Autodesk Inventor part; units mm, degrees
ref_plane "Work Plane1" through (0, 0, 10) normal (0, 0, 1) x (1, 0, 0)
ref_plane "YZ Plane" through (0, 0, 0) normal (1, 0, 0) x (0, 1, 0)
ref_plane "XZ Plane" through (0, 0, 0) normal (0, 1, 0) x (-1, 0, 0)
ref_plane "Work Plane1" through (0, 0, 10) normal (0, 0, 1) x (1, 0, 0)
sketch "Sketch1" plane through (0, 0, 10) normal (0, 0, 1) x (1, 0, 0)
  line L0 (-4.0299, -0.3538) -> (-2.2322, 1.4439) construction
  arc A0 (-1.4439, 2.2322) -> (-2.2322, 1.4439) centre (-0.9299, 0.9299) ccw construction
  line L1 (-1.4439, 2.2322) -> (0.3538, 4.0299) construction
  line L2 (-37.8299, 42.2137) -> (-37.8299, 45.8299) construction
  line L3 (-37.8299, 45.8299) -> (-4.0299, 45.8299) construction
  line L4 (-4.0299, 45.8299) -> (-4.0299, 42.2137) construction
  line L5 (-4.0299, 4.0299) -> (0.3538, 4.0299)
  circle A1 centre (-20.9299, 20.9299) radius 17.5 construction
  line L6 (-20.9299, 58.9723) -> (17.1124, 20.9299) construction
  line L7 (17.1124, 20.9299) -> (-20.9299, -17.1124) construction
  line L8 (-20.9299, -17.1124) -> (-58.9723, 20.9299) construction
  line L9 (-58.9723, 20.9299) -> (-20.9299, 58.9723) construction
  line L10 (-20.9299, 58.9723) -> (-20.9299, -17.1124) construction
  line L11 (17.1124, 20.9299) -> (-58.9723, 20.9299) construction
  line L12 (-20.9299, 58.9723) -> (32.8701, 58.9723) construction
  line L13 (-43.2198, 43.4299) -> (1.7802, 43.4299) construction
  line L14 (1.7802, 43.4299) -> (1.7802, -1.5701) construction
  line L15 (1.7802, -1.5701) -> (-43.2198, -1.5701) construction
  line L16 (-43.2198, -1.5701) -> (-43.2198, 43.4299) construction
  line L17 (-43.2198, 5.1774) -> (-43.2198, 36.6824)
  line L18 (-43.2198, 36.6824) -> (-36.4723, 43.4299)
  line L19 (-36.4723, 43.4299) -> (-5.3876, 43.4299)
  line L20 (-5.3876, 43.4299) -> (1.7802, 36.2621)
  line L21 (1.7802, 36.2621) -> (1.7802, 5.5977)
  line L22 (1.7802, 5.5977) -> (-5.3876, -1.5701)
  line L23 (-5.3876, -1.5701) -> (-36.4723, -1.5701)
  line L24 (-36.4723, -1.5701) -> (-43.2198, 5.1774)
  line L25 (-4.0299, 42.2137) -> (-37.8299, 42.2137)
  line L26 (-4.0299, -0.3538) -> (-4.0299, 4.0299)
  circle A2 centre (-20.7198, 20.9299) radius 7.0417 construction
  arc A3 (-7.3745, 3.5) -> (-34.4854, 3.5) centre (-20.9299, 0) ccw construction
  arc A4 (-11.4668, 9.7661) -> (-30.4087, 10.1422) centre (-20.7198, 20.9299) ccw
  line L27 (-30.5806, 10.1422) -> (-30.4087, 10.1422)
  line L28 (-30.4087, 10.1422) -> (-30.4087, 1.6029)
  line L29 (-30.4087, 1.6029) -> (-11.4668, 1.6029)
  line L30 (-11.4668, 1.6029) -> (-11.4668, 9.7661)
  line L31 (-43.2198, 43.4299) -> (-10.4667, 10.6769) construction
  line L32 (-8.5595, 8.5517) -> (1.7802, -1.5701) construction
  line L33 (1.7802, 43.4299) -> (-25.699, 15.9507) construction
  line L34 (-30.9728, 10.6769) -> (-43.2198, -1.5701) construction
  point P0 (-37.8299, 4.0299)
  dimension "d18" = 53.8
  dimension "d19" = 45
  dimension "d20" = 53.8
  dimension "d21" = 45
  dimension "d22" = 45
  dimension "d68" = 29
extrude "Extrusion1" add sketch "Sketch1" along normal blind 8
sketch "Sketch3" plane through (0, 0, 10) normal (0, 0, -1) x (-1, 0, 0)
  line L0 (37.8299, -0.4701) -> (37.8299, 4.0299) construction
  line L1 (4.0299, 4.0299) -> (4.0299, -0.4701) construction
  line L2 (37.8299, -0.4701) -> (37.8299, 1.1886) construction
  line L3 (4.0299, -3.9701) -> (4.0299, -0.3538) construction
  line L4 (45.8299, 4.0299) -> (42.2137, 4.0299) construction
  line L5 (-0.3538, 4.0299) -> (-3.9701, 4.0299) construction
  line L6 (-3.9701, 37.8299) -> (-0.3538, 37.8299) construction
  line L7 (4.0299, 42.2137) -> (4.0299, 45.8299) construction
  line L8 (37.8299, 45.8299) -> (37.8299, 42.2137) construction
  line L9 (42.2137, 37.8299) -> (45.8299, 37.8299) construction
  line L10 (37.8299, 37.7299) -> (45.8299, 37.7299)
  line L11 (45.8299, 37.7299) -> (45.8299, 4.1299)
  line L12 (45.8299, 4.1299) -> (37.8299, 4.1299)
  line L13 (37.8299, 4.1299) -> (37.8299, 37.7299)
  line L14 (37.7299, 4.0299) -> (4.1299, 4.0299)
  line L15 (4.1299, 4.0299) -> (4.1299, -3.9701)
  line L16 (4.1299, -3.9701) -> (37.7299, -3.9701)
  line L17 (37.7299, -3.9701) -> (37.7299, 4.0299)
  line L18 (4.0299, 4.1299) -> (-3.9701, 4.1299)
  line L19 (-3.9701, 4.1299) -> (-3.9701, 37.7299)
  line L20 (-3.9701, 37.7299) -> (4.0299, 37.7299)
  line L21 (4.0299, 37.7299) -> (4.0299, 4.1299)
  line L22 (4.1299, 37.8299) -> (37.7299, 37.8299)
  line L23 (37.7299, 37.8299) -> (37.7299, 45.8299)
  line L24 (37.7299, 45.8299) -> (4.1299, 45.8299)
  line L25 (4.1299, 45.8299) -> (4.1299, 37.8299)
  point P0 (0, 0)
  dimension "d23" = 0.1
  dimension "d24" = 0.1
  dimension "d25" = 0.1
  dimension "d26" = 0.1
  dimension "d27" = 0.1
extrude "Extrusion3" add sketch "Sketch3" against normal up to surface (8 mm away)
sketch "Skizze12" plane through (0, 0, 10) normal (0, 0, -1) x (-1, 0, 0)
  line L0 (-0.3124, 4.1299) -> (4.1299, -0.3124)
  line L1 (4.1299, -0.3124) -> (4.1299, -3.9701)
  line L2 (4.1299, -3.9701) -> (37.7299, -3.9701) construction
  line L3 (37.7299, -3.9701) -> (37.7299, -0.3124)
  line L4 (37.7299, -0.3124) -> (42.1723, 4.1299)
  line L5 (45.8299, 4.1299) -> (42.1723, 4.1299)
  line L6 (45.8299, 37.7299) -> (45.8299, 4.1299) construction
  line L7 (42.1723, 37.7299) -> (45.8299, 37.7299)
  line L8 (42.1723, 37.7299) -> (37.7299, 42.1723)
  line L9 (37.7299, 42.1723) -> (37.7299, 45.8299)
  line L10 (37.7299, 45.8299) -> (4.1299, 45.8299) construction
  line L11 (4.1299, 45.8299) -> (4.1299, 42.1723)
  line L12 (4.1299, 42.1723) -> (-0.3124, 37.7299)
  line L13 (-3.9701, 37.7299) -> (-0.3124, 37.7299)
  line L14 (-3.9701, 4.1299) -> (-3.9701, 37.7299) construction
  line L15 (-0.3124, 4.1299) -> (-3.9701, 4.1299)
  line L16 (37.9299, -4.1701) -> (3.9299, -4.1701) construction
  line L17 (3.9299, -4.1701) -> (3.9299, -0.3953)
  line L18 (3.9299, -0.3953) -> (-0.3953, 3.9299)
  line L19 (-0.3953, 3.9299) -> (-4.1701, 3.9299)
  line L20 (-4.1701, 3.9299) -> (-4.1701, 37.9299) construction
  line L21 (-4.1701, 37.9299) -> (-0.3953, 37.9299)
  line L22 (-0.3953, 37.9299) -> (3.9299, 42.2551)
  line L23 (3.9299, 42.2551) -> (3.9299, 46.0299)
  line L24 (3.9299, 46.0299) -> (37.9299, 46.0299) construction
  line L25 (37.9299, 46.0299) -> (37.9299, 42.2551)
  line L26 (37.9299, 42.2551) -> (42.2551, 37.9299)
  line L27 (42.2551, 37.9299) -> (46.0299, 37.9299)
  line L28 (46.0299, 37.9299) -> (46.0299, 3.9299) construction
  line L29 (46.0299, 3.9299) -> (42.2551, 3.9299)
  line L30 (42.2551, 3.9299) -> (37.9299, -0.3953)
  line L31 (37.9299, -0.3953) -> (37.9299, -4.1701)
  line L32 (-3.9701, 37.7299) -> (-3.9701, 37.9299)
  line L33 (37.7299, 45.8299) -> (4.1299, 45.8299)
  line L34 (4.1299, 45.8299) -> (3.9299, 45.8299)
  line L35 (37.7299, 45.8299) -> (37.9299, 45.8299)
  line L36 (45.8299, 37.7299) -> (45.8299, 37.9299)
  line L37 (45.8299, 4.1299) -> (45.8299, 3.9299)
  line L38 (37.7299, -3.9701) -> (37.9299, -3.9701)
  line L39 (4.1299, -3.9701) -> (3.9299, -3.9701)
  line L40 (-3.9701, 4.1299) -> (-3.9701, 3.9299)
  point P0 (0, 0)
  dimension "d65" = 0.2
extrude "IM_offset" add sketch "Skizze12" against normal up to surface (8 mm away)
sketch "Sketch14" plane through (0, 0, 10) normal (0, 0, -1) x (-1, 0, 0)
  arc A0 (5.5299, 0) -> (1.3299, 0) centre (3.4299, 0) ccw
  line L0 (37.8999, 16.97) -> (37.8999, -16.97)
  circle A1 centre (38.3947, 20.9299) radius 1.4
  circle A2 centre (3.4299, 0) radius 1.4
  point P0 (0, 0)
  dimension "d69" = 2.8
  dimension "d70" = 2.8
extrude "Extrusion12" cut sketch "Sketch14" against normal blind 10
properties part number "20_Cube_Insert_RaspiCam_v3"
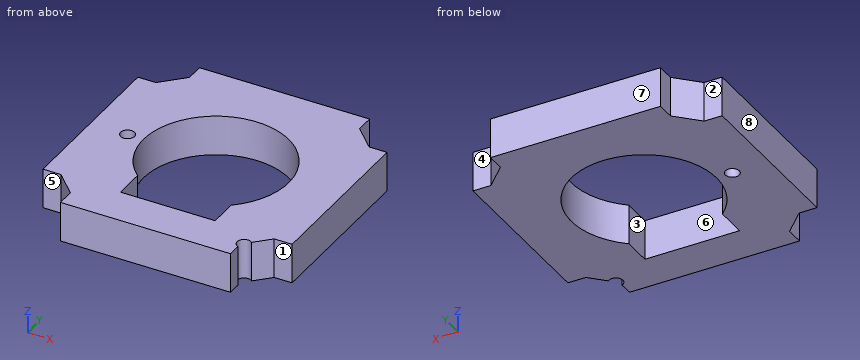
Could you check a few things on this model? Use its own coordinates, in mm. Face numbers are marked on the shaded views. A direction names the side the tool comes from. Coordinates: 2 decimals unless noted, no trailing zeros. Write each loop counter-clockwise with the first axis right and the second up, starting at its lowest first coordinate (ties: lowest second). Pieces come first, ordered by that corner, then holes. Notation, with made-up numbers: (20.5, 77) -> (70.5, 77) arc R13 cw to (70.5, 100) -> close; hole circle Ø1 at (74, 11). An arc over 180 degrees is marked (long way). Write item = value, one per line. Start each with the question number.
(1) I want a section at A-A (x = -25). Please give me the cut outline in (y, z).
(2) I want a section at C-C (z = 13). Please give me the cut outline in (x, y), plus the area to 3 significant figures.
(3) We'd pull the mould along Y, two halves only. Please class the marked faces 1, 2 and 3: released by +Y, released by -Y, zero draft, split by the parting line, or undercut.
(4) I need wall thicknesses on line 1 (X direction, y = 9.5, z = 15.25); line 2 (X direction, y = -1.5, z = 16.25); line 3 (Y direction, x = -39.5, z = 12.5) (3 decimals). Which ranges of each line are inside material? Lowest first, please. Write a range as [from, to].
(5) I want a section at B-B (y = 16.5). Please give me the cut outline in (x, z).
(6) Will these pins go through, and if not, where does the flat tip stop? pin 1 (0.8 mm diameter, centred on y = -3, z = 13, fed in from +X); pin 2 (4 mm diameter, centred on y = 45, z = 15.5, fed in from -X); pin 3 (1.1 mm diameter, centred on x = 2.5, z = 13.5, fed in from +Y).
(7) Which directions (+Z, -Z, +X, -X, +Y, -Y) give clear straight access to the entire face, cutting with the end or side of a thin tool? Please do the marked faces 4, 5, 6, 7 and 8.
Result set:
q1.outline = (-3.97, 10) -> (4.03, 10) -> (4.03, 18) -> (-3.97, 18) -> close; (34.78, 10) -> (45.83, 10) -> (45.83, 18) -> (34.78, 18) -> close
q2.outline = (-45.83, 3.93) -> (-42.26, 3.93) -> (-37.93, -0.4) -> (-37.93, -3.97) -> (-3.93, -3.97) -> (-3.93, -1.31) arc R1.4 cw (long way) to (-2.49, 1.04) -> (0.4, 3.93) -> (3.97, 3.93) -> (3.97, 37.93) -> (0.4, 37.93) -> (-3.93, 42.26) -> (-3.93, 45.83) -> (-37.93, 45.83) -> (-37.93, 42.26) -> (-42.26, 37.93) -> (-45.83, 37.93) -> close; hole circle Ø2.8 at (-38.39, 20.93); hole (-30.41, 4.03) -> (-11.47, 4.03) -> (-11.47, 9.77) arc R14.5 ccw (long way) to (-30.41, 10.14) -> close
q2.area = 1,530 mm2
q3.face_1 = released by -Y
q3.face_2 = released by +Y
q3.face_3 = undercut
q4.line_1 = [-45.83, -30.41], [-11.47, 3.97]
q4.line_2 = [-37.93, -3.93]
q4.line_3 = [1.175, 20.071], [21.789, 40.685]
q5.outline = (-45.83, 10) -> (-34.53, 10) -> (-34.53, 18) -> (-45.83, 18) -> close; (-6.91, 10) -> (3.97, 10) -> (3.97, 18) -> (-6.91, 18) -> close
q6.pin_1 = -3.93
q6.pin_2 = -37.93
q6.pin_3 = 37.93
q7.face_4 = +Z, -Z, +X, +Y
q7.face_5 = +Z, -Z, -X, -Y
q7.face_6 = +Z, -Z
q7.face_7 = +Z, -Z, +X, -X, +Y
q7.face_8 = +Z, -Z, -X, +Y, -Y
